For this review, use the dimensioned drawing (mm, ordinates from the lowest corner) and the shaded views. A direction names the side the tool comes from. Round coordinates to 2 decimals unless told otherwise and drop trailing zeros. Order: outer loops, then holes, each group sorted by start corner. A loop starts at its lowest first (then second) coordinate and runs counter-clockwise, first axis right, second up. Notation, with made-up numbers: (37, 66) -> (57, 66) arc R20 ccw to (57, 90) -> close; hole circle Ø7 at (-13.75, 29.5). An arc over 180 degrees is marked (long way). Answer in a Markdown table with one row per item.
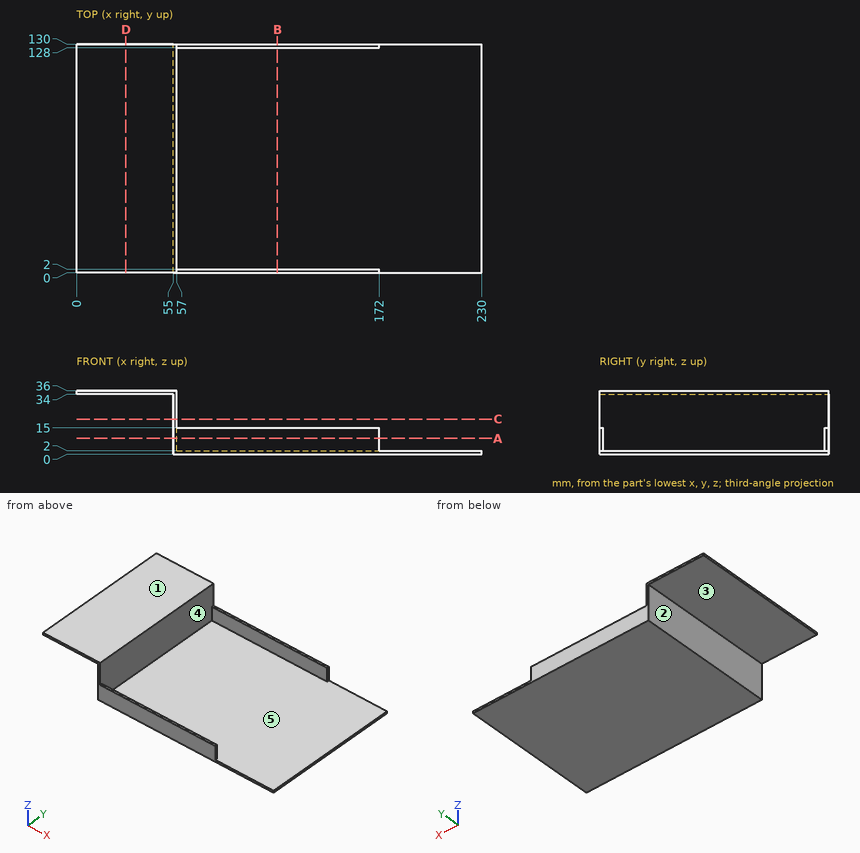
Q1. Take a section at D-D, the plane x = 28. Write out the cut boundary in (y, z), then the cut area to 3 significant figures.
Answer key:
| item | result |
|---|---|
| outline | (0, 34) -> (130, 34) -> (130, 36) -> (0, 36) -> close |
| area | 260 mm^2 |
Q2. Clearance check with flat-ended pins moving along their axes: pin 1 Ø1 at (y, z) = (129, 9.5) entering from +X; pin 2 Ø16.5 at (x, y) = (22, 86) entering from -Z; pin 3 Ø0.6 at (x, y) = (116.5, 1.5) entering from +Z. State where each tip first meets the part, or that it passes through.
Answer key:
| item | result |
|---|---|
| pin 1 | stops at x = 172 |
| pin 2 | stops at z = 34 |
| pin 3 | stops at z = 15 |
Q3. Take a section at B-B, the plane x = 114. Write out the cut boundary in (y, z), then the cut area to 3 significant figures.
Answer key:
| item | result |
|---|---|
| outline | (0, 0) -> (130, 0) -> (130, 15) -> (128, 15) -> (128, 2) -> (2, 2) -> (2, 15) -> (0, 15) -> close |
| area | 312 mm^2 |
Q4. Tool access review of the marked faces 1 and 2: name each direction out of +Z, -Z, +X, -X, +Y, -Y from which nothing blocks a thin tool from reaching the whole face with its end or side.
Answer key:
| item | result |
|---|---|
| face 1 | +Z, +X, -X, +Y, -Y |
| face 2 | -Z, -X, +Y, -Y |
Q5. To check wall thickness, follow probe 1 along Y at (x, z) = (156.5, 6); probe 2 along X at (y, z) = (27, 25.5); probe 3 along Z at (x, y) = (179, 27.5). State the ranges of each line that lie inside material, in increasing order.
Answer key:
| item | result |
|---|---|
| probe 1 | y = 0 to 2, 128 to 130 |
| probe 2 | x = 55 to 57 |
| probe 3 | z = 0 to 2 |
Q6. Take a section at C-C, the plane z = 20. Write out the cut boundary in (x, y), then the cut area to 3 significant figures.
Answer key:
| item | result |
|---|---|
| outline | (55, 0) -> (57, 0) -> (57, 130) -> (55, 130) -> close |
| area | 260 mm^2 |
Q7. The part is to be moulded in two halves that separate along Y. For the marked faces 3, 4 and 5, say which applies: +Y half, -Y half, draft (parallel to the pull), parting line (faces both ways), or undercut.
Answer key:
| item | result |
|---|---|
| face 3 | draft |
| face 4 | undercut |
| face 5 | undercut |
Q8. Take a section at A-A, the plane z = 9. Write out the cut boundary in (x, y).
Answer key:
| item | result |
|---|---|
| outline | (55, 0) -> (172, 0) -> (172, 2) -> (57, 2) -> (57, 128) -> (172, 128) -> (172, 130) -> (55, 130) -> close |
